The listing builds one solid part. Answer for the finished solid, in the listing's coordinates (mm). A direction names the side the tool comes from. Coordinates: 2 decimals unless noted, no trailing zeros. Write each loop counter-clockwise with the first axis right and the second up, starting at its lowest first coordinate (ties: lowest second). Pieces come first, ordered by that corner, then holes.
from build123d import *

# Parameters (mm, degrees)
F0_W     = 60
F0_H     = 15
F1_DEPTH = 5
F2_W     = 60
F2_H     = 5
F3_DEPTH = 10
F4_R     = 1.25
F4_R_2   = 1.3
F4_R_3   = 1.35
F4_R_4   = 1.4
F4_R_5   = 1.45
F4_R_6   = 1.5
F5_DEPTH = 5
F6_R     = 1.5
F6_R_2   = 1.45
F6_R_3   = 1.4
F6_R_4   = 1.35
F6_R_5   = 1.3
F6_R_6   = 1.25
F7_DEPTH = 5
F8_W     = 64
F8_H     = 19
F8_W_2   = 60
F8_H_2   = 15
F9_DEPTH = 0.2


with BuildPart() as f1:
    # F0 (on Top) → F1 (new body)
    with BuildSketch(Plane.XY):
        with Locations((30, 7.5)):
            Rectangle(F0_W, F0_H)
    extrude(amount=F1_DEPTH)

    # F2 (on face) → F3 (join)
    with BuildSketch(Plane.XY.offset(5)):
        with Locations((30, 2.5)):
            Rectangle(F2_W, F2_H)
    extrude(amount=F3_DEPTH)

    # F4 (on face) → F5 (cut, through all)
    with BuildSketch(Plane.XY.offset(5)):
        with Locations((5, 10)):
            Circle(F4_R)
        with Locations((15, 10)):
            Circle(F4_R_2)
        with Locations((25, 10)):
            Circle(F4_R_3)
        with Locations((35, 10)):
            Circle(F4_R_4)
        with Locations((45, 10)):
            Circle(F4_R_5)
        with Locations((55, 10)):
            Circle(F4_R_6)
    extrude(amount=-F5_DEPTH, mode=Mode.SUBTRACT)

    # F6 (on face) → F7 (cut, through all)
    with BuildSketch(Plane(origin=(0, 5, 0), x_dir=(-1, 0, 0), z_dir=(0, 1, 0))):
        with Locations((-55, 10)):
            Circle(F6_R)
        with Locations((-45, 10)):
            Circle(F6_R_2)
        with Locations((-35, 10)):
            Circle(F6_R_3)
        with Locations((-25, 10)):
            Circle(F6_R_4)
        with Locations((-15, 10)):
            Circle(F6_R_5)
        with Locations((-5, 10)):
            Circle(F6_R_6)
    extrude(amount=-F7_DEPTH, mode=Mode.SUBTRACT)

    # F8 (on Top) → F9 (join)
    with BuildSketch(Plane.XY):
        with Locations((30, 7.5)):
            Rectangle(F8_W, F8_H)
        with Locations((30, 7.5)):
            Rectangle(F8_W_2, F8_H_2, mode=Mode.SUBTRACT)
    extrude(amount=F9_DEPTH)


solid = f1.part
1. Section C-C on z = 10 is taken. Give the vertices of the cut face in (x, y), then the cut area to 4 significant figures.
Results found:
outline: (0, 0) - (3.75, 0) - (3.75, 5) - (0, 5) - close; (6.25, 0) - (13.7, 0) - (13.7, 5) - (6.25, 5) - close; (16.3, 0) - (23.65, 0) - (23.65, 5) - (16.3, 5) - close; (26.35, 0) - (33.6, 0) - (33.6, 5) - (26.35, 5) - close; (36.4, 0) - (43.55, 0) - (43.55, 5) - (36.4, 5) - close; (46.45, 0) - (53.5, 0) - (53.5, 5) - (46.45, 5) - close; (56.5, 0) - (60, 0) - (60, 5) - (56.5, 5) - close
area: 217.5 mm2
2. Find the intervals of material crossed by L1, parallel to Y at x = 55, z = 3.25; L2, parallel to Z at x = 15, y = 2.3, in increasing order.
Results found:
L1: y = 0 to 8.5, 11.5 to 15
L2: z = 0 to 8.7, 11.3 to 15
3. A tool of negligible diameter and unlimited length cuts with its end or side. For faces 5 (the flat face through (30, 10, 5)), 6 (the cylindrical face through (33.97, 10.95, 2.54)), 7 (the flat face through (30, 0, 7)), from which of +Z, -Z, +X, -X, +Y, -Y can it reach the whole face along a straight path? Write none if from no direction.
Results found:
face 5: +Z, +X, -X, +Y
face 6: +Z, -Z
face 7: +Z, +X, -X, -Y
4. Section A-A on x = 5 is taken. Give the vertices of the cut face in (y, z).
Results found:
outline: (-2, 0) - (8.75, 0) - (8.75, 5) - (5, 5) - (5, 8.75) - (0, 8.75) - (0, 0.2) - (-2, 0.2) - close; (0, 11.25) - (5, 11.25) - (5, 15) - (0, 15) - close; (11.25, 0) - (17, 0) - (17, 0.2) - (15, 0.2) - (15, 5) - (11.25, 5) - close
5. Flat-ended cylindrical pins translate along their axes: P1, Ø5, axis at x = 29, z = 12, coming from the +Y side; P2, Ø5, axis at x = 55, z = 10, coming from the -Y side; P3, Ø3, axis at x = 15, y = 10, coming from the -Z side; P4, Ø6, axis at x = 30.5, y = 14, coming from the +Z side. Find the tip coordinate at first contact, or state that the pin passes through.
Results found:
P1: stops at y = 5
P2: stops at y = 0
P3: stops at z = 0
P4: stops at z = 5
6. Section B-B on y = 10 is taken. State how many separate pieces and enclosed holes the cut face has, then the cut area to 3 significant figures.
Results found:
separate pieces: 7
enclosed holes: 0
area: 218 mm2
7. For a pull along X with two mould halves and no side action, classify faces 1 (the flat face through (30, 5, 10)), 2 (the flat face through (60, 6, 4)), 3 (the cylindrical face through (56.43, 10.45, 2.54)), 4 (the flat face through (0, 6, 4)) as pulls with the +X half, pulls with the -X half, needs draft (parallel to the pull), parting line crosses it, or undercut.
Results found:
face 1: needs draft
face 2: pulls with the +X half
face 3: undercut
face 4: pulls with the -X half
8. Section D-D on z = 3.75 is taken. Give the vertices of the cut face in (x, y).
Results found:
outline: (0, 0) - (60, 0) - (60, 15) - (0, 15) - close; hole circle Ø2.5 at (5, 10); hole circle Ø2.6 at (15, 10); hole circle Ø2.7 at (25, 10); hole circle Ø2.8 at (35, 10); hole circle Ø2.9 at (45, 10); hole circle Ø3 at (55, 10)
